Drawing for the job (mm, zero at the part's lowest x, y, z). Give positions to 0.01 mm unless a question says otherwise; leave off trailing zeros. Order: outer loops, then holes, each group sorted by start corner. A loop starts at its lowest first (then second) coordinate and runs counter-clockwise, first axis right, second up. Notation, with made-up numbers: M 24.5,39.5 L 82.5,39.5 A6 ccw 82.5,49.5 Z; hole C -27.5,36.5 d8. An arc over 180 degrees is marked long. One line per item, written item: value.
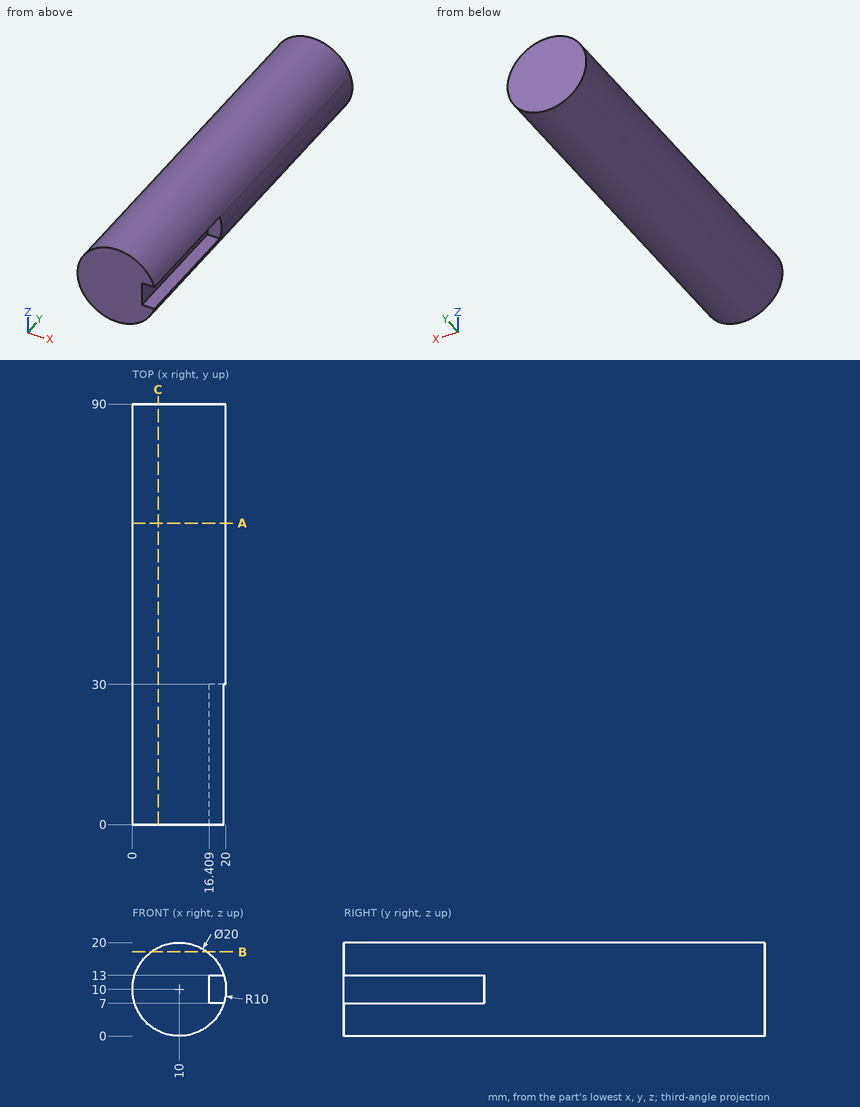
1) Saw through at A-A, the plane y = 64.5. Write the cut outline in (x, z).
Check values:
outline: C 10,10 d20
2) Pin check, flat tips, straight feed: pin 1 (3 mm diameter, centred on x = 14.5, z = 15, fed in from -Y); pin 2 (3 mm diameter, centred on x = 6, y = 58.5, fed in from -Z); pin 3 (1.8 mm diameter, centred on x = 18, z = 11, fed in from -Y); pin 4 (2 mm diameter, centred on y = 37, z = 15.5, fed in from +X). Stop position of each tip, or through.
Check values:
pin 1: y = 0
pin 2: z = 0.32
pin 3: y = 30
pin 4: x = 18.93
3) Saw through at B-B, the plane z = 18. Write the cut outline in (x, y), then the cut area to 3 significant figures.
Check values:
outline: M 4,0 L 16,0 L 16,90 L 4,90 Z
area: 1,080 mm^2
4) Drill centre lines: probe 1 along Z at (x, y) = (10, 8.5); probe 2 along X at (y, z) = (42, 12.75) (1 decimal); probe 3 along Z at (x, y) = (8.5, 66). Where is each one in solid material? Low to high. Write a range as from..to.
Check values:
probe 1: 0..20
probe 2: 0.4..19.6
probe 3: 0.11..19.89
5) Saw through at C-C, the plane x = 5.5. Write the cut outline in (y, z).
Check values:
outline: M 0,1.07 L 90,1.07 L 90,18.93 L 0,18.93 Z
